from build123d import *

# Parameters (mm, degrees)
SKETCH1_W           = 50
SKETCH1_H           = 21
BOSS_EXTRUDE1_DEPTH = 58
SKETCH3_R           = 7.5
CUT_EXTRUDE1_DEPTH  = 24
CUT_EXTRUDE2_REACH  = 66.025
SKETCH4_R           = 5
CUT_EXTRUDE3_START  = -24
SKETCH5_R           = 7.5
CUT_EXTRUDE3_DEPTH  = 24
CUT_EXTRUDE4_REACH  = 66.025
SKETCH6_R           = 4.5
CUT_EXTRUDE5_REACH  = 68.558
SKETCH8_W           = 10
SKETCH8_H           = 18
SKETCH7_R           = 4.1
CUT_EXTRUDE6_DEPTH  = 15


with BuildPart() as part:
    # Sketch1 → Boss-Extrude1 (new body)
    with BuildSketch(Plane(origin=(0, 0, 0), x_dir=(1, 0, 0), z_dir=(0, 1, 0))):
        Rectangle(SKETCH1_W, SKETCH1_H)
    extrude(amount=BOSS_EXTRUDE1_DEPTH)

    # Sketch3 → Cut-Extrude1 (cut)
    with BuildSketch(Plane(origin=(0, 58, 0), x_dir=(1, 0, 0), z_dir=(0, 1, 0))):
        with Locations(Location((-15, 0, 0), (0, 0, 270))):
            Circle(SKETCH3_R)
    extrude(amount=-CUT_EXTRUDE1_DEPTH, mode=Mode.SUBTRACT)

    # Sketch4 → Cut-Extrude2 (cut, up to next)
    with BuildSketch(Plane(origin=(0, 58, 0), x_dir=(1, 0, 0), z_dir=(0, 1, 0)), mode=Mode.PRIVATE) as cut_extrude2_sk1:
        with Locations(Location((15, 0, 0), (0, 0, 270))):
            Circle(SKETCH4_R)
    cut_extrude2_tool1 = extrude(cut_extrude2_sk1.sketch, amount=-CUT_EXTRUDE2_REACH, mode=Mode.PRIVATE) & part.part
    add(cut_extrude2_tool1.solids().sort_by_distance((15, 58, 0))[0], mode=Mode.SUBTRACT)

    # Sketch5 → Cut-Extrude3 (cut)
    with BuildSketch(Plane.XZ.offset(CUT_EXTRUDE3_START)):
        with Locations(Location((-15, 0, 0), (0, 0, 90))):
            Circle(SKETCH5_R)
    extrude(amount=CUT_EXTRUDE3_DEPTH, mode=Mode.SUBTRACT)

    # Sketch6 → Cut-Extrude4 (cut, up to next)
    with BuildSketch(Plane.XZ, mode=Mode.PRIVATE) as cut_extrude4_sk1:
        with Locations(Location((-15, 0, 0), (0, 0, 270))):
            Circle(SKETCH6_R)
    cut_extrude4_tool1 = extrude(cut_extrude4_sk1.sketch, amount=-CUT_EXTRUDE4_REACH, mode=Mode.PRIVATE) & part.part
    add(cut_extrude4_tool1.solids().sort_by_distance((-15, 0, 0))[0], mode=Mode.SUBTRACT)

    # Sketch8 → Cut-Extrude5 (cut, up to next)
    with BuildSketch(Plane.XY.offset(10.5), mode=Mode.PRIVATE) as cut_extrude5_sk1:
        with Locations((0, 29)):
            Rectangle(SKETCH8_W, SKETCH8_H)
    cut_extrude5_tool1 = extrude(cut_extrude5_sk1.sketch, amount=-CUT_EXTRUDE5_REACH, mode=Mode.PRIVATE) & part.part
    add(cut_extrude5_tool1.solids().sort_by_distance((0, 29, 10.5))[0], mode=Mode.SUBTRACT)

    # Sketch7 → Cut-Extrude6 (cut)
    with BuildSketch(Plane.XY.offset(10.5)):
        with Locations((0, 46)):
            Circle(SKETCH7_R)
        with Locations(Location((0, 12, 0), (0, 0, 180))):
            Circle(SKETCH7_R)
    extrude(amount=-CUT_EXTRUDE6_DEPTH, mode=Mode.SUBTRACT)


solid = part.part
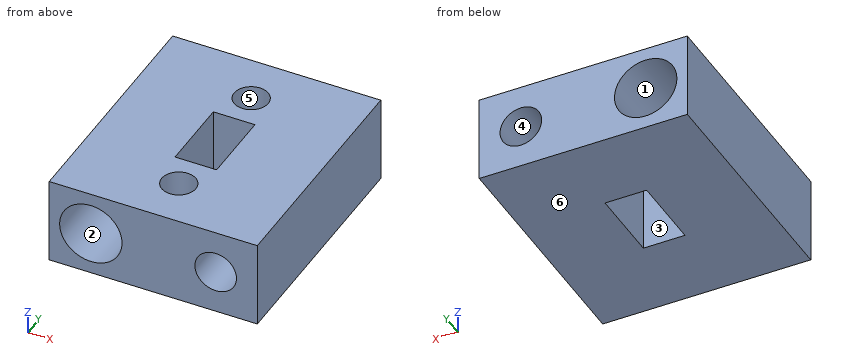
Geometry: final body of the model. Coordinates: model frame, mm. Face numbers are marked on the shaded views. A direction names the side the tool comes from. Coordinates: 2 decimals unless noted, no trailing zeros. Write each loop counter-clockwise with the first axis right and the second up, starting at its lowest first coordinate (ties: lowest second). Pieces come first, ordered by that corner, then holes. Notation, with made-up numbers: (33.5, 80) - (47.5, 80) arc R28 cw to (47.5, 115) - close; hole circle Ø3 at (16.25, 83). An arc over 180 degrees is marked (long way). Return JSON: item names as keys, results as strings.
Item 1: Section query C-C (x = 0). Output: boundary loops of the cut face in (y, z).
Completed:
{"outline": "(0, -10.5) - (20, -10.5) - (20, 10.5) - (16.1, 10.5) - (16.1, -4.5) - (7.9, -4.5) - (7.9, 10.5) - (0, 10.5) - close; (38, -10.5) - (58, -10.5) - (58, 10.5) - (50.1, 10.5) - (50.1, -4.5) - (41.9, -4.5) - (41.9, 10.5) - (38, 10.5) - close"}
Item 2: Line query: L1, parallel to X at y = 53, z = 0.25; L2, parallel to Y at x = -3, z = 4.25; L3, parallel to X at y = 43.5, z = 6.75. Output: solid intervals per line, ascending.
Completed:
{"L1": "x = -25 to -22.5, -7.5 to 10.01, 19.99 to 25", "L2": "y = 0 to 9.21, 14.79 to 20, 38 to 43.21, 48.79 to 58", "L3": "x = -25 to -18.27, -11.73 to -3.25, 3.25 to 25"}
Item 3: Pull-direction query (Z, two-part tool) for the marked faces 4, 5 and 6; classes: +Z half, -Z half, draft (parallel to the pull), parting line (faces both ways), or undercut.
Completed:
{"face 4": "undercut", "face 5": "draft", "face 6": "-Z half"}
Item 4: Reachability of the marked faces 1, 2 and 3 from +Z, -Z, +X, -X, +Y, -Y: full face, straight path, thin tool, end or side. Return the list, or none.
Completed:
{"face 1": "+Y", "face 2": "-Y", "face 3": "+Z, -Z"}
Item 5: Section query B-B (y = 31.5). Output: boundary loops of the cut face in (x, z), and give its area (3 significant figures).
Completed:
{"outline": "(-25, -10.5) - (-5, -10.5) - (-5, 10.5) - (-25, 10.5) - close; (5, -10.5) - (25, -10.5) - (25, 10.5) - (5, 10.5) - close; hole circle Ø9 at (-15, 0); hole circle Ø10 at (15, 0)", "area": "698 mm2"}
Item 6: Section query D-D (y = 53). Output: boundary loops of the cut face in (x, z).
Completed:
{"outline": "(-25, -10.5) - (25, -10.5) - (25, 10.5) - (-25, 10.5) - close; hole circle Ø15 at (-15, 0); hole circle Ø10 at (15, 0)"}
Item 7: Pin query (flat end, axial travel): pin 1 Ø5 at (x, y) = (0, 12) entering from +Z; pin 2 Ø5.5 at (x, z) = (-15, 0) entering from +Y. Return the tip coordinate at first contact, or that it passes through.
Completed:
{"pin 1": "stops at z = -4.5", "pin 2": "passes through"}
Item 8: Section query A-A (z = 0). Output: boundary loops of the cut face in (x, y), and give its area (3 significant figures).
Completed:
{"outline": "(-25, 0) - (-22.5, 0) - (-22.5, 24) - (-19.5, 24) - (-19.5, 34) - (-22.5, 34) - (-22.5, 58) - (-25, 58) - close; (-10.5, 24) - (-7.5, 24) - (-7.5, 0) - (10, 0) - (10, 58) - (-7.5, 58) - (-7.5, 34) - (-10.5, 34) - close; (20, 0) - (25, 0) - (25, 58) - (20, 58) - close; hole (-5, 20) - (5, 20) - (5, 38) - (-5, 38) - close; hole circle Ø8.2 at (0, 12); hole circle Ø8.2 at (0, 46)", "area": "1,220 mm2"}
